Here's how the part is built. I have some questions about the finished solid (model axes, mm). Face numbers are marked on the shaded views. A direction names the side the tool comes from. Give positions to 0.01 mm unless a question says otherwise; leave off trailing zeros. Loops run counter-clockwise (first coordinate to the right, second up) from the corner with the lowest first, then second, coordinate; pieces in that order, holes last.
Q1. If we section it at B-B (y = 0): Please give me the cut outline in (x, z).
Q2. If we section it at D-D (z = 33.5): Please give me the cut outline in (x, y), plus the area to 3 significant figures.
Q3. I need wall thicknesses on line 1 (Y direction, x = 50, z = 13.25); line 2 (X direction, y = -19.5, z = 30); line 3 (Z direction, x = 41, y = -9). Which ranges of each line are inside material? Lowest first, please.
Q4. If we section it at A-A (z = 4): Please give me the cut outline in (x, y).
Q5. For the marked faces 1, 2 and 3, which set-ups out of +Z, -Z, +X, -X, +Y, -Y let a thin tool reach every point of the face, with its end or its side?
Q6. We'd pull the mould along Y, two halves only. Please class the marked faces 4, 5, 6 and 7: +Y half, -Y half, draft (parallel to the pull), parting line (faces both ways), or undercut.
Q7. Will these pins go through, and if not, where does the flat tip stop? P1, Ø3, axis at y = -20.5, z = 18.5, coming from the -X side; P2, Ø4, axis at x = 17.5, y = -17, coming from the -Z side; P3, Ø4, axis at x = -7.5, y = -14, coming from the +Z side.
Q8. If we section it at C-C (x = 51): Please give me the cut outline in (y, z).
from build123d import *

# Parameters (mm, degrees)
F0_W     = 60
F0_H     = 6
F0_W_2   = 40
F1_DEPTH = 8
F2_DEPTH = 12
F0_R     = 5
F3_DEPTH = 24
F4_DEPTH = 36


with BuildPart() as f1:
    # F0 (on Top) → F1 (new body)
    with BuildSketch(Plane.XY):
        with Locations((0, -28)):
            Rectangle(F0_W, F0_H)
        with Locations((50, -28)):
            Rectangle(F0_W_2, F0_H)
        with Locations((0, 28)):
            Rectangle(F0_W, F0_H)
        with Locations((50, 28)):
            Rectangle(F0_W_2, F0_H)
    extrude(amount=-F1_DEPTH)

    # F0 (on Top) → F2 (join)
    with BuildSketch(Plane.XY):
        with Locations((0, 28)):
            Rectangle(F0_W, F0_H)
        Polygon((30, 25), (-30, 25), (-30, -25), (30, -25), (30, -18.5), (30, 18.5), align=None)
        with BuildLine():
            ThreePointArc((-10, -8), (-18, 0), (-10, 8))
            Line((-10, 8), (10, 8))
            ThreePointArc((10, 8), (18, 0), (10, -8))
            Line((10, -8), (-10, -8))
        make_face(mode=Mode.SUBTRACT)
        with Locations((0, -28)):
            Rectangle(F0_W, F0_H)
    extrude(amount=F2_DEPTH)

    # F0 (on Top) → F3 (join)
    with BuildSketch(Plane.XY):
        with Locations((50, 28)):
            Rectangle(F0_W_2, F0_H)
        Polygon((70, 25), (30, 25), (30, 18.5), (70, 12.5), align=None)
        Polygon((70, 12.5), (30, 18.5), (30, -18.5), (70, -12.5), align=None)
        with Locations((50, 0)):
            Circle(F0_R, mode=Mode.SUBTRACT)
        Polygon((30, -18.5), (30, -25), (70, -25), (70, -12.5), align=None)
        with Locations((50, -28)):
            Rectangle(F0_W_2, F0_H)
    extrude(amount=F3_DEPTH)

    # F0 (on Top) → F4 (join)
    with BuildSketch(Plane.XY):
        Polygon((30, -18.5), (30, -25), (70, -25), (70, -12.5), align=None)
        with Locations((50, -28)):
            Rectangle(F0_W_2, F0_H)
        Polygon((70, 25), (30, 25), (30, 18.5), (70, 12.5), align=None)
        with Locations((50, 28)):
            Rectangle(F0_W_2, F0_H)
    extrude(amount=F4_DEPTH)


solid = f1.part
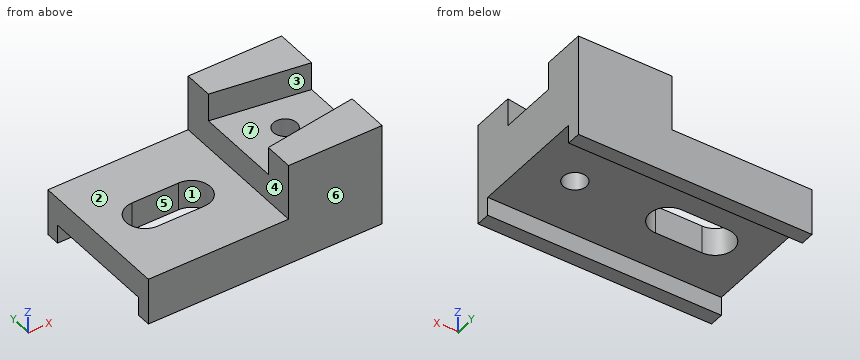
Check sheet entries:
1. outline: (-30, 0) - (-18, 0) - (-18, 12) - (-30, 12) - close; (18, 0) - (45, 0) - (45, 24) - (30, 24) - (30, 12) - (18, 12) - close; (55, 0) - (70, 0) - (70, 24) - (55, 24) - close
2. outline: (30, -31) - (70, -31) - (70, -12.5) - (30, -18.5) - close; (30, 18.5) - (70, 12.5) - (70, 31) - (30, 31) - close
2. area: 1,240 mm2
3. line 1: y = -31 to -5, 5 to 31
3. line 2: x = 30 to 70
3. line 3: z = 0 to 24
4. outline: (-30, -31) - (70, -31) - (70, 31) - (-30, 31) - close; hole (-10, -8) - (10, -8) arc R8 ccw to (10, 8) - (-10, 8) arc R8 ccw to start; hole circle Ø10 at (50, 0)
5. face 1: +Z, -Z
5. face 2: +Z, -X, +Y, -Y
5. face 3: +Z, -X
6. face 4: draft
6. face 5: undercut
6. face 6: -Y half
6. face 7: undercut
7. P1: stops at x = 30
7. P2: stops at z = 0
7. P3: stops at z = 12
8. outline: (-31, -8) - (-25, -8) - (-25, 0) - (-4.9, 0) - (-4.9, 24) - (-15.35, 24) - (-15.35, 36) - (-31, 36) - close; (4.9, 0) - (25, 0) - (25, -8) - (31, -8) - (31, 36) - (15.35, 36) - (15.35, 24) - (4.9, 24) - close
